Part model, mm, in its own coordinate system. A direction names the side the tool comes from. Give positions to 0.01 mm unless a question says otherwise; leave off trailing zeros. Write each loop counter-clockwise with the first axis right and the second up, starting at its lowest first coordinate (ties: lowest second). Pieces come first, ordered by that corner, then holes. Notation, with made-up numbers: M -26,-40 L 33,-40 A27 ccw 33,-17 Z; hole C 17.5,30 d11. An arc over 180 degrees is marked long. Use CSV: the item, a comma, the result in double quotes. Start each with the question number.
Item 1: Which spindle directions (+Z, -Z, +X, -X, +Y, -Y) get a long thin tool onto all of the face, cutting with end or side? Do faces 4 (the flat face through (-14, 10, 4)), 5 (the cylindrical face through (2.01, -9.03, 7.39)). Say none if no direction does.
Item 2: Mould opens along X. For faces 1 (the flat face through (-20, 0, 7)), 2 (the flat face through (0, 20, 7)), 3 (the cylindrical face through (10.381, -5.21, 5.492)) say: released by +X, released by -X, zero draft, split by the parting line, or undercut.
Item 3: Drill centre lines: line 1 (Z direction, x = 13, y = 15); line 2 (Z direction, x = 13, y = -1); line 3 (Y direction, x = 0, z = 9). Where is each one in solid material? Low to high. Write a range as [from, to].
Item 4: Pin check, flat tip, straight feed: pin 1 (5 mm diameter, centred on x = 14.5, z = 6, fed in from +Y). Stop position of the tip, or through.
Item 5: Cut at B-B (z = 7.5). List the corners of the cut face in (x, y).
Item 6: Cut at C-C (x = -13). List the corners of the cut face in (y, z), then the cut area to 3 significant figures.
Item 7: Cut at A-A (y = 0). List the corners of the cut face in (x, z).
Item 8: Cut at D-D (x = 17). List the corners of the cut face in (y, z), then the cut area to 3 significant figures.
from build123d import *

# Parameters (mm, degrees)
SKETCH_4_W                   = 40
SKETCH_4_H                   = 40
EXTRUDE_2_DEPTH              = 15
M20X1_5_2_D                  = 18.5
M20X1_5_2_DEPTH              = 44.5
M20X1_5_2_TIP                = 5.557960726
HOLE_WIZARD_M6_1_D           = 6.6
HOLE_WIZARD_M6_1_CBORE_D     = 10
HOLE_WIZARD_M6_1_CBORE_DEPTH = 10


with BuildPart() as part:
    # 草图4 → 凸台-拉伸2 (new body)
    with BuildSketch(Plane.XY):
        Rectangle(SKETCH_4_W, SKETCH_4_H)
    extrude(amount=EXTRUDE_2_DEPTH)

    # M20x1.5 螺纹孔2
    with Locations(Plane.XY.offset(15)):
        with Locations((0, 0)):
            Hole(M20X1_5_2_D / 2, depth=M20X1_5_2_DEPTH)
            with Locations((0, 0, -(M20X1_5_2_DEPTH + M20X1_5_2_TIP / 2))):  # 118° drill point
                Cone(0, M20X1_5_2_D / 2, M20X1_5_2_TIP, mode=Mode.SUBTRACT)

    # M6 凹头盖螺钉的柱形沉头孔1 (through all)
    with Locations(Plane(origin=(0, 20, 0), x_dir=(-1, 0, 0), z_dir=(0, 1, 0))):
        with Locations((13, 7.5), (-13, 7.5)):
            CounterBoreHole(HOLE_WIZARD_M6_1_D / 2, HOLE_WIZARD_M6_1_CBORE_D / 2, HOLE_WIZARD_M6_1_CBORE_DEPTH)


solid = part.part
Worked answers:
1,face 4,"+Y"
1,face 5,"+Z, -Z"
2,face 1,"released by -X"
2,face 2,"zero draft"
2,face 3,"undercut"
3,line 1,"z = [0, 2.5], [12.5, 15]"
3,line 2,"z = [0, 4.2], [10.8, 15]"
3,line 3,"y = [-20, -9.25], [9.25, 20]"
4,pin 1,"stops at y = 10"
5,outline,"M -20,-20 L -16.3,-20 L -16.3,10 L -18,10 L -18,20 L -20,20 Z; M -9.7,-20 L 9.7,-20 L 9.7,10 L 8,10 L 8,20 L -8,20 L -8,10 L -9.7,10 Z; M 16.3,-20 L 20,-20 L 20,20 L 18,20 L 18,10 L 16.3,10 Z; hole C 0,0 d18.5"
6,outline,"M -20,0 L 20,0 L 20,2.5 L 10,2.5 L 10,4.2 L -20,4.2 Z; M -20,10.8 L 10,10.8 L 10,12.5 L 20,12.5 L 20,15 L -20,15 Z"
6,area,"302 mm^2"
7,outline,"M -20,0 L -9.25,0 L -9.25,15 L -20,15 Z; M 9.25,0 L 20,0 L 20,15 L 9.25,15 Z; hole C -13,7.5 d6.6; hole C 13,7.5 d6.6"
8,outline,"M -20,0 L 20,0 L 20,4.5 L 10,4.5 L 10,10.5 L 20,10.5 L 20,15 L -20,15 Z"
8,area,"540 mm^2"
